The model under review builds one solid part; all positions refer to its coordinate system, in mm. Give positions to 0.01 mm unless a question says otherwise; leave off trailing zeros. Loops run counter-clockwise (first coordinate to the right, second up) from the corner with the lowest first, then second, coordinate; pieces in that order, holes last. Notation, with made-up numbers: M 51.25,53 L 105.25,53 A34 ccw 105.25,91 Z; hole C 10.25,-28.5 d3. An arc over 180 degrees is marked long. Return JSON: item names as keys, results as strings.
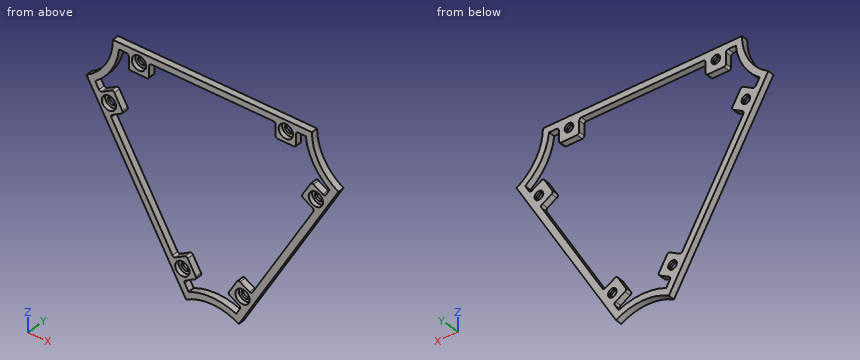
```python
from build123d import *

# Parameters (mm, degrees)
BOSS_EXTRUDE2_DEPTH = 3
SKETCH3_R           = 2.0000000000000036
SKETCH3_R_2         = 1.9999999999999967
SKETCH3_R_3         = 2.0000000000000027
SKETCH3_R_4         = 2.0000000000000018
CUT_EXTRUDE1_DEPTH  = 84.32734015621716
FILLET2_R           = 1
SKETCH5_R           = 3.299999999999997
SKETCH5_R_2         = 3.3000000000000003
SKETCH5_R_3         = 3.2999999999998377
CUT_EXTRUDE3_DEPTH  = 2


with BuildPart() as part:
    # Sketch2 → Boss-Extrude2 (new body)
    with BuildSketch(Plane(origin=(0, 0, 0), x_dir=(1, 0, 0), z_dir=(0, 1, 0))):
        with BuildLine():
            Line((-57.900347822426866, -19.41320198612938), (-45.90034782242687, 1.3714077046971502))
            Line((-45.90034782242687, 1.3714077046971502), (-24.137847822426874, 39.065163404414825))
            Line((-24.137847822426874, 39.065163404414825), (-12.137847822426867, 59.849773095241346))
            ThreePointArc((-12.137847822426867, 59.849773095241346), (-2.0632e-13, 56.59744657337059), (12.137847822426314, 59.849773095241474))
            Line((12.137847822426314, 59.849773095241474), (24.13784782242651, 39.06516340441507))
            Line((24.13784782242651, 39.06516340441507), (45.90034782242685, 1.3714077046975783))
            Line((45.90034782242685, 1.3714077046975783), (57.90034782242704, -19.413201986128836))
            ThreePointArc((57.90034782242704, -19.413201986128836), (49.014826521872, -28.298723286684716), (45.76250000000075, -40.43657110911115))
            Line((45.76250000000075, -40.43657110911115), (21.762500000000745, -40.43657110911158))
            Line((21.762500000000745, -40.43657110911158), (-21.762499999999243, -40.436571109112386))
            Line((-21.762499999999243, -40.436571109112386), (-45.762499999999235, -40.43657110911281))
            ThreePointArc((-45.762499999999235, -40.43657110911281), (-49.01482652187049, -28.298723286685338), (-57.900347822426866, -19.41320198612938))
        make_face()
        with BuildLine():
            Line((11.82759378458235, 40.3871488520415), (11.32759378458234, 41.25317425582594))
            Line((11.32759378458234, 41.25317425582594), (7.1275937845823325, 48.52778764761524))
            Line((7.1275937845823325, 48.52778764761524), (13.189771611073091, 52.02778764761513))
            Line((13.189771611073091, 52.02778764761513), (10.95702958785254, 55.895010272027164))
            ThreePointArc((10.95702958785254, 55.895010272027164), (-3.1e-14, 53.59744657337001), (-10.95702958785254, 55.895010272027164))
            Line((-10.95702958785254, 55.895010272027164), (-13.189771611074285, 52.0277876476148))
            Line((-13.189771611074285, 52.0277876476148), (-7.127593784582693, 48.52778764761462))
            Line((-7.127593784582693, 48.52778764761462), (-11.327593784582492, 41.25317425582568))
            Line((-11.327593784582492, 41.25317425582568), (-11.827593784582703, 40.38714885204087))
            Line((-11.827593784582703, 40.38714885204087), (-17.889771611074185, 43.88714885204099))
            Line((-17.889771611074185, 43.88714885204099), (-21.53977161107411, 37.56516340441455))
            Line((-21.53977161107411, 37.56516340441455), (-43.30227161107358, -0.12859229530344518))
            Line((-43.30227161107358, -0.12859229530344518), (-46.95227161107352, -6.450577742929913))
            Line((-46.95227161107352, -6.450577742929913), (-40.890093784582575, -9.950577742929706))
            Line((-40.890093784582575, -9.950577742929706), (-45.59009378458257, -18.091216538503463))
            Line((-45.59009378458257, -18.091216538503463), (-51.65227161107341, -14.591216538503707))
            Line((-51.65227161107341, -14.591216538503707), (-53.88501363429374, -18.458439162915578))
            ThreePointArc((-53.88501363429374, -18.458439162915578), (-46.4167503105172, -26.798723286685323), (-42.92798404644063, -37.43657110911222))
            Line((-42.92798404644063, -37.43657110911222), (-38.46249999999932, -37.436571109112705))
            Line((-38.46249999999932, -37.436571109112705), (-38.46249999999945, -30.436571109112176))
            Line((-38.46249999999945, -30.436571109112176), (-30.062499999999865, -30.436571109112133))
            Line((-30.062499999999865, -30.436571109112133), (-29.062499999999424, -30.43657110911213))
            Line((-29.062499999999424, -30.43657110911213), (-29.062499999999286, -37.43657110911253))
            Line((-29.062499999999286, -37.43657110911253), (-21.762499999999292, -37.43657110911241))
            Line((-21.762499999999292, -37.43657110911241), (21.762500000000696, -37.4365711091116))
            Line((21.762500000000696, -37.4365711091116), (29.062500000000714, -37.436571109111476))
            Line((29.062500000000714, -37.436571109111476), (29.062500000000565, -30.436571109111707))
            Line((29.062500000000565, -30.436571109111707), (38.46250000000059, -30.436571109111636))
            Line((38.46250000000059, -30.436571109111636), (38.46250000000072, -37.436571109111306))
            Line((38.46250000000072, -37.436571109111306), (42.927984046442106, -37.43657110911252))
            ThreePointArc((42.927984046442106, -37.43657110911252), (46.41675031051867, -26.798723286684776), (53.88501363429554, -18.458439162914214))
            Line((53.88501363429554, -18.458439162914214), (51.65227161107371, -14.591216538502506))
            Line((51.65227161107371, -14.591216538502506), (45.59009378458266, -18.09121653850257))
            Line((45.59009378458266, -18.09121653850257), (40.890093784582604, -9.950577742928846))
            Line((40.890093784582604, -9.950577742928846), (46.95227161107361, -6.450577742928804))
            Line((46.95227161107361, -6.450577742928804), (43.30227161107357, -0.12859229530243052))
            Line((43.30227161107357, -0.12859229530243052), (21.539771611073228, 37.565163404415046))
            Line((21.539771611073228, 37.565163404415046), (17.88977161107317, 43.88714885204144))
            Line((17.88977161107317, 43.88714885204144), (11.82759378458235, 40.3871488520415))
        make_face(mode=Mode.SUBTRACT)
    extrude(amount=BOSS_EXTRUDE2_DEPTH)

    # Sketch3 → Cut-Extrude1 (cut, through all)
    with BuildSketch(Plane(origin=(0, 3, 0), x_dir=(1, 0, 0), z_dir=(0, 1, 0))):
        with Locations(Location((33.762500000000074, -35.45259651289613, 0), (0, 0, 270))):
            Circle(SKETCH3_R)
        with Locations(Location((-33.76249999999959, -35.45259651289661, 0), (0, 0, 270))):
            Circle(SKETCH3_R_2)
        with Locations(Location((-47.58409921028776, -11.5128844388239, 0), (0, 0, 270))):
            Circle(SKETCH3_R_3)
        with Locations(Location((47.58409921028791, -11.512884438823233, 0), (0, 0, 270))):
            Circle(SKETCH3_R_3)
        with Locations(Location((13.821599210288047, 46.96548095172012, 0), (0, 0, 270))):
            Circle(SKETCH3_R)
        with Locations(Location((-13.821599210288047, 46.96548095172012, 0), (0, 0, 270))):
            Circle(SKETCH3_R_4)
    extrude(amount=-CUT_EXTRUDE1_DEPTH, mode=Mode.SUBTRACT)

    # Fillet2
    fillet2_edges = [part.edges().sort_by_distance(p)[0] for p in [
        (-46.95227161107352, 1.5, 6.450577742929913),
        (-40.890093784582575, 1.5, 9.950577742929706),
        (-45.59009378458257, 1.5, 18.091216538503463),
        (-51.65227161107341, 1.5, 14.591216538503707),
        (-38.46249999999932, 1.5, 37.436571109112705),
        (-38.46249999999945, 1.5, 30.436571109112176),
        (-29.062499999999424, 1.5, 30.43657110911213),
        (-29.062499999999286, 1.5, 37.43657110911253),
        (29.062500000000714, 1.5, 37.436571109111476),
        (29.062500000000565, 1.5, 30.436571109111707),
        (38.46250000000059, 1.5, 30.436571109111636),
        (38.46250000000072, 1.5, 37.436571109111306),
        (51.65227161107371, 1.5, 14.591216538502506),
        (45.59009378458266, 1.5, 18.09121653850257),
        (40.890093784582604, 1.5, 9.950577742928846),
        (46.95227161107361, 1.5, 6.450577742928804),
        (17.88977161107317, 1.5, -43.88714885204144),
        (11.82759378458235, 1.5, -40.3871488520415),
        (7.1275937845823325, 1.5, -48.52778764761524),
        (13.189771611073091, 1.5, -52.02778764761513),
        (-13.189771611074285, 1.5, -52.0277876476148),
        (-7.127593784582693, 1.5, -48.52778764761462),
        (-11.827593784582703, 1.5, -40.38714885204087),
        (-17.889771611074185, 1.5, -43.88714885204099),
    ]]
    fillet(fillet2_edges, radius=FILLET2_R)

    # Sketch5 → Cut-Extrude3 (cut)
    with BuildSketch(Plane.XZ):
        with Locations(Location((47.58409921028791, 11.512884438823233, 0), (0, 0, 270))):
            Circle(SKETCH5_R)
        with Locations(Location((33.762500000000074, 35.45259651289613, 0), (0, 0, 270))):
            Circle(SKETCH5_R)
        with Locations(Location((-13.821599210288472, -46.96548095172, 0), (0, 0, 270))):
            Circle(SKETCH5_R_2)
        with Locations(Location((13.821599210287625, -46.96548095172023, 0), (0, 0, 270))):
            Circle(SKETCH5_R_2)
        with Locations(Location((-33.76249999999945, 35.45259651289674, 0), (0, 0, 270))):
            Circle(SKETCH5_R)
        with Locations(Location((-47.5840992102877, 11.512884438824086, 0), (0, 0, 270))):
            Circle(SKETCH5_R_3)
    extrude(amount=-CUT_EXTRUDE3_DEPTH, mode=Mode.SUBTRACT)


solid = part.part
```
1) Consider section B-B on z = -24. Write out the cut boundary in (x, y), then the cut area to 3 significant figures.
From the geometry:
{"outline": "M -32.84,0 L -29.37,0 L -29.37,3 L -32.84,3 Z; M 29.37,0 L 32.84,0 L 32.84,3 L 29.37,3 Z", "area": "20.8 mm²"}
2) Consider section A-A on x = -4. Write out the cut boundary in (y, z).
From the geometry:
{"outline": "M 0,-56.93 L 3,-56.93 L 3,-53.89 L 0,-53.89 Z; M 0,37.44 L 3,37.44 L 3,40.44 L 0,40.44 Z"}
3) Consider section C-C on y = 1.2. Count the separate pieces of the cut face and the enclosed holes in it, then the cut area to 3 significant figures.
From the geometry:
{"separate pieces": "1", "enclosed holes": "7", "area": "1,200 mm²"}
4) Insertion check: pin 1 (0.9 mm diameter, centred on x = -5, y = 1, fed in from -Z); pin 2 (6 mm diameter, centred on x = -33.76, z = 35.45, fed in from -Y); pin 3 (1.5 mm diameter, centred on y = 1, z = -10.5, fed in from +X); pin 4 (3.5 mm diameter, centred on x = -47.58, z = 11.51, fed in from +Y). Each pin has a flat end and moves straight along its axis. Give the tip position at first contact, or say it passes through.
From the geometry:
{"pin 1": "z = -57.22", "pin 2": "y = 2", "pin 3": "x = 41.06", "pin 4": "through"}
5) Wall thickness on L1, parallel to Z at x = 11, y = 0.85; L2, parallel to Z at x = 14, y = 1.4; L3, parallel to X at y = 1.45, z = -47: over which ranges is each line inside the solid? List them lowest first. Write a range as from..to.
From the geometry:
{"L1": "-59.23..-55.82, -50.76..-48.68, -45.25..-41.82, 37.44..40.44", "L2": "-56.62..-50.26, -43.67..-41.64, 37.44..40.44", "L3": "-19.56..-17.12, -10.52..-8.01, 8.01..10.52, 17.12..19.56"}
